Check sheet for the modelled part. Datum: model origin and axes. Units: mm. Face numbers are marked on the shaded views. A direction names the side the tool comes from. Give positions to 0.01 mm unless a question says otherwise; leave off trailing zeros. Order: outer loops, then holes, each group sorted by start corner. A loop starts at its lowest first (then second) coordinate and runs counter-clockwise, first axis right, second up.
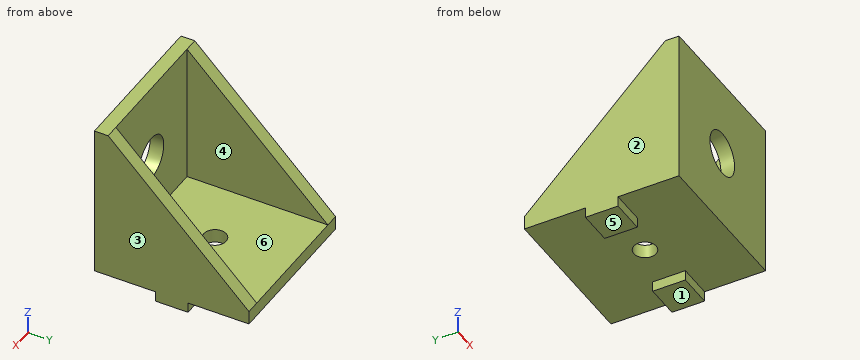
Autodesk Fusion 360 part; units mm, degrees
sketch "Sketch1" plane through (0, 0, 0) normal (0, 1, 0) x (1, 0, 0)
  line L0 (22.5, 22.5) -> (-22.5, 22.5)
  line L1 (-22.5, 22.5) -> (-22.5, -22.5)
  line L2 (-22.5, -22.5) -> (22.5, -22.5)
  line L3 (22.5, -22.5) -> (22.5, 22.5)
  line L4 (22.5, 22.5) -> (-22.5, -22.5) construction
  line L5 (-22.5, 22.5) -> (22.5, -22.5) construction
  dimension "d1" = 45
  dimension "d2" = 45
extrude "Extrude1" add sketch "Sketch1" along normal blind 4
sketch "Sketch2" plane through (0, 0, -22.5) normal (0, 0, -1) x (-1, 0, 0)
  line L0 (22.5, 0) -> (-22.5, 0)
  line L1 (-22.5, 0) -> (-22.5, 45)
  line L2 (-22.5, 45) -> (22.5, 45)
  line L3 (22.5, 45) -> (22.5, 0)
  point P0 (-22.5, 0)
  point P1 (22.5, 0)
  dimension "d12" = 45
extrude "Extrude4" add sketch "Sketch2" against normal blind 4
sketch "Sketch3" plane through (-22.5, 0, 0) normal (-1, 0, 0) x (0, 0, 1)
  line L0 (-22.5, 0) -> (22.5, 0)
  line L1 (22.5, 0) -> (22.5, 4)
  line L2 (22.5, 4) -> (-18.5, 4)
  line L3 (-22.5, 45) -> (-22.5, 0)
  line L4 (-18.5, 45) -> (-18.5, 4)
  line L5 (22.5, 4) -> (-18.5, 45)
  line L6 (-18.5, 4) -> (-18.5, 45)
  line L7 (-18.5, 45) -> (-22.5, 45)
extrude "Extrude3" add sketch "Sketch3" against normal blind 4 contours L2 L4 L5 L6
mirror "Mirror1" about plane through (0, 0, 0) normal (1, 0, 0) of "Extrude3"
sketch "Sketch6" plane through (0, 0, -22.5) normal (0, 0, -1) x (-1, 0, 0)
  line L0 (-22.5, 0) -> (22.5, 0)
  line L1 (22.5, 0) -> (22.5, 45)
  line L2 (22.5, 45) -> (-22.5, 45)
  line L3 (-22.5, 45) -> (-22.5, 0)
  line L4 (22.5, 27.25) -> (-22.5, 27.25)
  line L5 (-22.5, 27.25) -> (-22.5, 17.75)
  line L6 (-22.5, 17.75) -> (22.5, 17.75)
  line L7 (22.5, 17.75) -> (22.5, 27.25)
  line L8 (22.5, 27.25) -> (-22.5, 17.75) construction
  line L9 (-22.5, 27.25) -> (22.5, 17.75) construction
  line L10 (0, 0) -> (0, 6.5) construction
  line L11 (12.5, 27.25) -> (-12.5, 27.25)
  line L12 (-12.5, 27.25) -> (-12.5, 17.75)
  line L13 (-12.5, 17.75) -> (12.5, 17.75)
  line L14 (12.5, 17.75) -> (12.5, 27.25)
  line L15 (12.5, 27.25) -> (-12.5, 17.75) construction
  line L16 (-12.5, 27.25) -> (12.5, 17.75) construction
  point P0 (0, 22.5)
  point P1 (0, 22.5)
  dimension "d31" = 9.5
  dimension "d32" = 22.5
  dimension "d35" = 25
extrude "Extrude7" add sketch "Sketch6" along normal blind 3 contours L3 L4 L5 L6 L12 | L1 L4 L6 L7 L14
sketch "Sketch4" plane through (0, 0, -18.5) normal (0, 0, 1) x (1, 0, 0)
  line L0 (18.5, 45) -> (-18.5, 45)
  line L1 (-18.5, 45) -> (-18.5, 4)
  line L2 (-18.5, 4) -> (18.5, 4)
  line L3 (22.5, 45) -> (-22.5, 45)
  line L4 (-22.5, 0) -> (22.5, 0)
  line L5 (0, 0) -> (0, 20.1593) construction
  circle A0 centre (0, 22.5) radius 3.25
  dimension "d29" = 6.5
  dimension "d30" = 22.5
extrude "Extrude5" cut sketch "Sketch4" against normal through all
sketch "Sketch5" plane through (0, 0, 0) normal (0, -1, 0) x (1, 0, 0)
  line L0 (22.5, -22.5) -> (22.5, 22.5)
  line L1 (-22.5, 22.5) -> (-22.5, -22.5)
  line L2 (-22.5, -22.5) -> (22.5, -22.5)
  line L3 (-22.5, -22.5) -> (22.5, -22.5)
  circle A0 centre (0, 0) radius 6.4
  dimension "d28" = 12.8
extrude "Extrude6" cut sketch "Sketch5" against normal blind 4
equation "d30 = ( 45 / 2 ) * 1 mm"
equation "d32 = ( 45 / 2 ) * 1 mm"
1) Material ranges on L1, parallel to X at y = 21.5, z = -5; L2, parallel to Z at x = 0, y = 3; L3, parallel to Z at x = 15, y = 17.5, recorded low to high.
Recorded:
L1: x = -22.5 to -18.5, 18.5 to 22.5
L2: z = -22.5 to -6.4, 6.4 to 22.5
L3: z = -22.5 to -18.5
2) Set-up check for the marked faces 5 and 6: record each of +Z, -Z, +X, -X, +Y, -Y from which the full face is reachable in a straight line by a thin tool's end or side.
Recorded:
face 5: -Z, +X, -X, +Y, -Y
face 6: +Z, +Y
3) Section check B-B, the plane y = 22.5. Record the cut outline in (x, z), then the cut area to 3 significant figures.
Recorded:
outline: (-22.5, -25.5) - (-12.5, -25.5) - (-12.5, -22.5) - (-3.25, -22.5) - (-3.25, -18.5) - (-18.5, -18.5) - (-18.5, 4) - (-22.5, 4) - close; (3.25, -22.5) - (12.5, -22.5) - (12.5, -25.5) - (22.5, -25.5) - (22.5, 4) - (18.5, 4) - (18.5, -18.5) - (3.25, -18.5) - close
area: 394 mm2
4) Draft check along X on the marked faces 1, 2, 3 and 4. Enter one of: +X half, -X half, draft (parallel to the pull), parting line (faces both ways), or undercut.
Recorded:
face 1: draft
face 2: -X half
face 3: +X half
face 4: undercut
5) Section check C-C, the plane z = 0. Record the cut outline in (x, y).
Recorded:
outline: (-22.5, 0) - (-6.4, 0) - (-6.4, 4) - (-18.5, 4) - (-18.5, 26.5) - (-22.5, 26.5) - close; (6.4, 0) - (22.5, 0) - (22.5, 26.5) - (18.5, 26.5) - (18.5, 4) - (6.4, 4) - close
6) Section check D-D, the plane y = 12. Record the cut outline in (x, z), then the cut area to 3 significant figures.
Recorded:
outline: (-22.5, -22.5) - (22.5, -22.5) - (22.5, 14.5) - (18.5, 14.5) - (18.5, -18.5) - (-18.5, -18.5) - (-18.5, 14.5) - (-22.5, 14.5) - close
area: 444 mm2
7) Depth check by flat-ended pin: pin 1 Ø4 at (x, z) = (11, 6) entering from +Y; pin 2 Ø10 at (x, y) = (-9.5, 23.5) entering from +Z; pin 3 Ø7.5 at (x, z) = (0, 0) entering from +Y; pin 4 Ø0.9 at (x, z) = (-16.5, -24) entering from -Y. Enter the tip coordinate at first touch or a pass-through.
Recorded:
pin 1: stops at y = 4
pin 2: stops at z = -18.5
pin 3: passes through
pin 4: stops at y = 17.75
8) Section check A-A, the plane x = 0. Record the cut outline in (y, z).
Recorded:
outline: (0, -22.5) - (19.25, -22.5) - (19.25, -18.5) - (4, -18.5) - (4, -6.4) - (0, -6.4) - close; (0, 6.4) - (4, 6.4) - (4, 22.5) - (0, 22.5) - close; (25.75, -22.5) - (45, -22.5) - (45, -18.5) - (25.75, -18.5) - close
